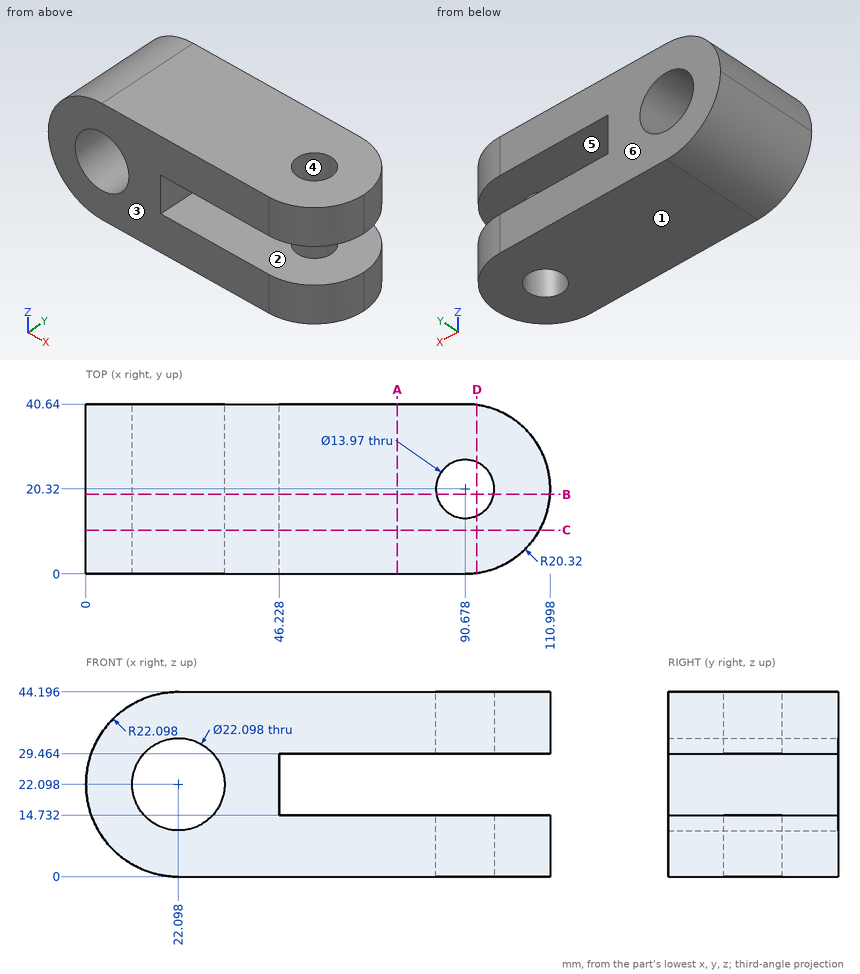
Geometry: see drawing. Coordinates: mm, zero at the bounding-box minimum. A direction names the side the tool comes from. Round coordinates to 2 decimals unless told otherwise and drop trailing zeros. Loops run counter-clockwise (first coordinate to the right, second up) from the corner with the lowest first, then second, coordinate; pieces in that order, holes last. Notation, with made-up numbers: M 63.5,-3 L 71.5,-3 A17 ccw 71.5,30 Z; hole C 26,10 d1. An arc over 180 degrees is marked long. Use a Markdown table: item, result. Add a question column.
1. Contact query for flat-ended pins moving along their axis: pin 1 (16 mm diameter, centred on y = 29.5, z = 22.5, fed in from +X); pin 2 (4 mm diameter, centred on y = 25, z = 15, fed in from -X); pin 3 (12 mm diameter, centred on y = 6.5, z = 37, fed in from -X). Output: stop coordinate, or through.
2. Cut plane D-D, the plane x = 93.5. Output: boundary loops of the cut face in (y, z), and give its area (3 significant figures).
3. Cut plane C-C, the plane y = 10.5. Output: boundary loops of the cut face in (x, z).
4. Cut plane A-A, the plane x = 74.5. Output: boundary loops of the cut face in (y, z), and give its area (3 significant figures).
5. Pull-direction query (Y, two-part tool) for the marked faces 3, 4, 5 and 6; classes: +Y half, -Y half, draft (parallel to the pull), parting line (faces both ways), or undercut.
6. Set-up query: the marked faces 1 and 2. Return all of +Z, -Z, +X, -X, +Y, -Y with unobstructed straight access to the full face (end or side cutting, diameter ignored); none if empty.
7. Cut plane B-B, the plane y = 19. Output: boundary loops of the cut face in (x, z), and give its area (3 significant figures).
8. Ray query, line 1 along Z through (x, y) = (100, 33); line 2 along X through (y, z) = (36, 22); line 3 along X through (y, z) = (15, 14.5). Return the intervals inside material, ascending. Write a range as [from, to].
Solution:
| question | item | result |
|---|---|---|
| 1 | pin 1 | stops at x = 110.31 |
| 1 | pin 2 | stops at x = 0.6 |
| 1 | pin 3 | stops at x = 1.87 |
| 2 | outline | M 0.2,0 L 13.93,0 L 13.93,14.73 L 0.2,14.73 Z; M 0.2,29.46 L 13.93,29.46 L 13.93,44.2 L 0.2,44.2 Z; M 26.71,0 L 40.44,0 L 40.44,14.73 L 26.71,14.73 Z; M 26.71,29.46 L 40.44,29.46 L 40.44,44.2 L 26.71,44.2 Z |
| 2 | area | 809 mm2 |
| 3 | outline | M 22.1,0 L 108.47,0 L 108.47,14.73 L 46.23,14.73 L 46.23,29.46 L 108.47,29.46 L 108.47,44.2 L 22.1,44.2 A22.1 ccw Z; hole C 22.1,22.1 d22.1 |
| 4 | outline | M 0,0 L 40.64,0 L 40.64,14.73 L 0,14.73 Z; M 0,29.46 L 40.64,29.46 L 40.64,44.2 L 0,44.2 Z |
| 4 | area | 1,200 mm2 |
| 5 | face 3 | -Y half |
| 5 | face 4 | undercut |
| 5 | face 5 | draft |
| 5 | face 6 | +Y half |
| 6 | face 1 | -Z, +X, -X, +Y, -Y |
| 6 | face 2 | +X, +Y, -Y |
| 7 | outline | M 22.1,0 L 83.82,0 L 83.82,14.73 L 46.23,14.73 L 46.23,29.46 L 83.82,29.46 L 83.82,44.2 L 22.1,44.2 A22.1 ccw Z; M 97.54,0 L 110.96,0 L 110.96,14.73 L 97.54,14.73 Z; M 97.54,29.46 L 110.96,29.46 L 110.96,44.2 L 97.54,44.2 Z; hole C 22.1,22.1 d22.1 |
| 7 | area | 2,950 mm2 |
| 8 | line 1 | z = [0, 14.73], [29.46, 44.2] |
| 8 | line 2 | x = [0, 11.05], [33.15, 46.23] |
| 8 | line 3 | x = [1.35, 14.08], [30.12, 86.15], [95.2, 110.29] |
